Part model, mm, in its own coordinate system. A direction names the side the tool comes from. Round coordinates to 2 decimals unless told otherwise and drop trailing zeros. Loops run counter-clockwise (first coordinate to the right, second up) from the corner with the lowest first, then second, coordinate; pieces in that order, holes last.
(1) Tool access for faces 3 (the face through (-3.246, -5.234, 0.23)), 4 (the face through (-3.5, -4, -2)), 5 (the face through (3.254, -5.234, 0.23)): list every direction of +Z, -Z, +X, -X, +Y, -Y with a clear straight run to the whole face (end or side of a thin tool).
(2) Mould opens along Y. For faces 1 (the face through (-3, 4, -4)), 2 (the face through (-3.5, 0, 10)) say: +Y half, -Y half, draft (parallel to the pull), parting line (faces both ways), or undercut.
(3) Cut at C-C on x = 2. List the corners of the cut face in (y, z), then the cut area to 3 significant figures.
(4) Flat gauge pins, fed straight in: pin 1 (1.5 mm diameter, centred on y = 7.5, z = -3.5, fed in from -X); pin 2 (5 mm diameter, centred on y = 0, z = 0, fed in from -X); pin 3 (3 mm diameter, centred on x = -1, z = 3, fed in from -Y); pin 4 (1 mm diameter, centred on y = 4.5, z = 4, fed in from +X). Where does each tip first touch, or does it go through?
(5) Cut at A-A on z = 0. List the corners of the cut face in (x, y), then the cut area to 3 significant figures.
(6) Probe probe 1 along Z at (x, y) = (-3.2, 0); probe 2 along Z at (x, y) = (-1.25, 0); probe 3 along X at (y, z) = (0.75, 7.5). List the from-to ranges inside material, lowest first.
(7) Cut at D-D on y = 5.5. List the corners of the cut face in (x, z), then the cut area to 3 significant figures.
from build123d import *

# Parameters (mm, degrees)
F0_R     = 11
F0_R_2   = 4
F1_DEPTH = 3
F2_R     = 11
F2_R_2   = 9.5415407764
F2_R_3   = 5.2393235044
F2_R_4   = 4
F3_DEPTH = 3.5


with BuildPart() as f1:
    # F0 (on Right) → F1 (new body, symmetric)
    with BuildSketch(Plane.YZ):
        Circle(F0_R)
        Circle(F0_R_2, mode=Mode.SUBTRACT)
    extrude(amount=F1_DEPTH, both=True)

    # F2 (on Right) → F3 (join, symmetric)
    with BuildSketch(Plane.YZ):
        Circle(F2_R)
        Circle(F2_R_2, mode=Mode.SUBTRACT)
        Circle(F2_R_3)
        Circle(F2_R_4, mode=Mode.SUBTRACT)
    extrude(amount=F3_DEPTH, both=True)


solid = f1.part
Final values:
1. face 3: -X
1. face 4: +Z, -Z, -X, +Y, -Y
1. face 5: +X
2. face 1: undercut
2. face 2: draft
3. outline: circle Ø22 at (0, 0); hole circle Ø8 at (0, 0)
3. area: 330 mm2
4. pin 1: stops at x = -3
4. pin 2: passes through
4. pin 3: stops at y = -10.9
4. pin 4: stops at x = 3
5. outline: (-3.5, -11) - (3.5, -11) - (3.5, -9.54) - (3, -9.54) - (3, -5.24) - (3.5, -5.24) - (3.5, -4) - (-3.5, -4) - (-3.5, -5.24) - (-3, -5.24) - (-3, -9.54) - (-3.5, -9.54) - close; (-3.5, 4) - (3.5, 4) - (3.5, 5.24) - (3, 5.24) - (3, 9.54) - (3.5, 9.54) - (3.5, 11) - (-3.5, 11) - (-3.5, 9.54) - (-3, 9.54) - (-3, 5.24) - (-3.5, 5.24) - close
5. area: 89.4 mm2
6. probe 1: z = -11 to -9.54, -5.24 to -4, 4 to 5.24, 9.54 to 11
6. probe 2: z = -11 to -4, 4 to 11
6. probe 3: x = -3 to 3
7. outline: (-3.5, -9.53) - (3.5, -9.53) - (3.5, -7.8) - (3, -7.8) - (3, 7.8) - (3.5, 7.8) - (3.5, 9.53) - (-3.5, 9.53) - (-3.5, 7.8) - (-3, 7.8) - (-3, -7.8) - (-3.5, -7.8) - close
7. area: 118 mm2
